from build123d import *

# Parameters (mm, degrees)
SKETCH_1_W          = 25
SKETCH_1_H          = 25
EXTRUDE_1_DEPTH     = 10
SKETCH_2_W          = 12.5
SKETCH_2_H          = 12.5
CUT_EXTRUDE_1_DEPTH = 21.310096012
SKETCH_3_W          = 25
SKETCH_3_H          = 25
EXTRUDE_2_DEPTH     = 5
SKETCH_4_R          = 2
CUT_EXTRUDE_2_DEPTH = 24.184046239
SKETCH_5_W          = 15
SKETCH_5_H          = 40
EXTRUDE_3_DEPTH     = 3
SKETCH_9_W          = 30
SKETCH_9_H          = 10
EXTRUDE_7_DEPTH     = 3
SKETCH_11_R         = 1.5
CUT_EXTRUDE_3_DEPTH = 50.749371855
EXTRUDE_8_DEPTH     = 12.5
EXTRUDE_9_DEPTH     = 3
SKETCH_15_R         = 1.25
CUT_EXTRUDE_4_DEPTH = 10
EXTRUDE_START       = -3
EXTRUDE_10_DEPTH    = 3


# Read off the part's stored shape, not the designer's step: 凸台-拉伸10
with BuildPart() as part:
    # 草图1 → 凸台-拉伸1 (new body)
    with BuildSketch(Plane.XY):
        Rectangle(SKETCH_1_W, SKETCH_1_H)
    extrude(amount=EXTRUDE_1_DEPTH)

    # 草图2 → 切除-拉伸1 (cut, through all)
    with BuildSketch(Plane.XY.offset(10)):
        Rectangle(SKETCH_2_W, SKETCH_2_H)
    extrude(amount=-CUT_EXTRUDE_1_DEPTH, mode=Mode.SUBTRACT)

    # 草图3 → 凸台-拉伸2 (add)
    with BuildSketch(Plane.XY.offset(10)):
        Rectangle(SKETCH_3_W, SKETCH_3_H)
    extrude(amount=EXTRUDE_2_DEPTH)

    # 草图4 → 切除-拉伸2 (cut, through all)
    with BuildSketch(Plane.XY.offset(15)):
        Circle(SKETCH_4_R)
    extrude(amount=-CUT_EXTRUDE_2_DEPTH, mode=Mode.SUBTRACT)

    # 草图5 → 凸台-拉伸3 (add)
    with BuildSketch(Plane(origin=(-12.5, 12.5, 0), x_dir=(0, 0, -1), z_dir=(0.7071067811865477, -0.7071067811865474, 0))):
        with Locations((-20, 0)):
            Rectangle(SKETCH_5_W, SKETCH_5_H)
    extrude(amount=EXTRUDE_3_DEPTH)

    # 草图9 → 凸台-拉伸7 (add)
    with BuildSketch(Plane(origin=(-10.378679656, 10.378679656, 0), x_dir=(0, 0, -1), z_dir=(0.7071067811865477, -0.7071067811865474, 0))):
        with Locations((-20, 25)):
            Rectangle(SKETCH_9_W, SKETCH_9_H)
    extrude_7 = extrude(amount=-EXTRUDE_7_DEPTH)

    # 草图11 → 切除-拉伸3 (cut, through all)
    with BuildSketch(Plane(origin=(-12.5, 12.5, 0), x_dir=(0, 0, 1), z_dir=(-0.7071067811865477, 0.7071067811865474, 0))):
        with Locations(Location((11, 24, 0), (0, 0, 270))):
            Circle(SKETCH_11_R)
        with Locations(Location((29, 24, 0), (0, 0, 270))):
            Circle(SKETCH_11_R)
    cut_extrude_3 = extrude(amount=-CUT_EXTRUDE_3_DEPTH, mode=Mode.SUBTRACT)

    # 草图12 → 凸台-拉伸8 (add)
    with BuildSketch(Plane(origin=(0, 0, 12.5), x_dir=(-1, 0, 0), z_dir=(0, 0, -1))):
        Polygon((8.257359313, 12.5), (12.5, 8.257359313), (14.621320344, 10.378679656), (10.378679656, 14.621320344), align=None)
    extrude(amount=EXTRUDE_8_DEPTH)

    # 草图13 → 凸台-拉伸9 (add)
    with BuildSketch(Plane(origin=(12.5, 12.5, 0), x_dir=(0, 0, -1), z_dir=(-0.7071067811865474, -0.7071067811865477, 0))):
        with BuildLine():
            Line((-27.5, -14.67766953), (-12.5, -14.67766953))
            ThreePointArc((-12.5, -14.67766953), (-3.210155108, -9.92766953), (0, 0))
            Line((0, 0), (-15, 0))
            ThreePointArc((-15, 0), (-18.349852274, -9.808698696), (-27.5, -14.67766953))
        make_face()
    extrude_9 = extrude(amount=EXTRUDE_9_DEPTH)

    # 草图15 → 切除-拉伸4 (cut)
    with BuildSketch(Plane(origin=(12.5, 0, 0), x_dir=(0, 0, -1), z_dir=(1, 0, 0))):
        with Locations(Location((-7.5, 0, 0), (0, 0, 90))):
            Circle(SKETCH_15_R)
    cut_extrude_4 = extrude(amount=-CUT_EXTRUDE_4_DEPTH, mode=Mode.SUBTRACT)

    # 凸台-拉伸10 outline → 凸台-拉伸10 (add)
    with BuildSketch(Plane(origin=(12.5, 12.5, 0), x_dir=(0, 0, -1), z_dir=(0.7071067811865474, 0.7071067811865477, 0)).offset(EXTRUDE_START)):
        with BuildLine():
            ThreePointArc((-12.5, 14.67766953), (-3.949281056, 10.728388475), (0, 2.177669532))
            Line((0, 2.177669532), (0, 17.67766953))
            Line((0, 17.67766953), (-12.5, 17.67766953))
            Line((-12.5, 17.67766953), (-12.5, 14.67766953))
        make_face()
    extrude_10 = extrude(amount=EXTRUDE_10_DEPTH)

    # 镜向3: 凸台-拉伸7, 切除-拉伸3, 凸台-拉伸9, 切除-拉伸4, 凸台-拉伸10 across plane
    add(extrude_7.mirror(Plane(origin=(0, 0, 0), x_dir=(0, 0, 1), z_dir=(-0.7071067811865474, -0.7071067811865477, 0))))
    add(cut_extrude_3.mirror(Plane(origin=(0, 0, 0), x_dir=(0, 0, 1), z_dir=(-0.7071067811865474, -0.7071067811865477, 0))), mode=Mode.SUBTRACT)
    add(extrude_9.mirror(Plane(origin=(0, 0, 0), x_dir=(0, 0, 1), z_dir=(-0.7071067811865474, -0.7071067811865477, 0))))
    add(cut_extrude_4.mirror(Plane(origin=(0, 0, 0), x_dir=(0, 0, 1), z_dir=(-0.7071067811865474, -0.7071067811865477, 0))), mode=Mode.SUBTRACT)
    add(extrude_10.mirror(Plane(origin=(0, 0, 0), x_dir=(0, 0, 1), z_dir=(-0.7071067811865474, -0.7071067811865477, 0))))


solid = part.part
Check sheet for the modelled part. Datum: model origin and axes. Units: mm. A direction names the side the tool comes from. Round coordinates to 2 decimals unless told otherwise and drop trailing zeros. Loops run counter-clockwise (first coordinate to the right, second up) from the corner with the lowest first, then second, coordinate; pieces in that order, holes last. Notation, with made-up numbers: (33, 79.25) - (68, 79.25) arc R30 cw to (68, 113.25) - close; hole circle Ø1 at (20.25, -31). An arc over 180 degrees is marked (long way). Answer as CSV lines item,"result". Start each with the question number.
Item 1: Release check for a two-part mould opening along Z. For faces 6 (the cylindrical face through (-12.235, -10.673, -0.044)), 7 (the flat face through (6.54, 27.3, 20.21)), 8 (the cylindrical face through (9.42, -0.27, 6.28)), 9 (the flat face through (-29, -6, 35)) record: +Z half, -Z half, draft (parallel to the pull), parting line (faces both ways), or undercut.
Item 2: Section check D-D (x = -23.5). Record the boundary of the cut face in (y, z), and give its area (3 significant figures).
Item 3: Set-up check for faces 1 (the flat face through (-32.638, -9.789, 20.21)), 2 (the flat face through (-27.3, -6.54, 20.21)), 3 (the flat face through (-25.567, -2.718, 8.802)), 4 (the flat face through (2.718, 25.567, 31.302)), 5 (the flat face through (-25.567, -2.718, 31.302)): record each of +Z, -Z, +X, -X, +Y, -Y from which the full face is reachable in a straight line by a thin tool's end or side.
Item 4: Scan lines: line 1 (X direction, y = -2.5, z = 13); line 2 (Y direction, x = -0.5, z = 11.5); line 3 (X direction, y = -10.75, z = 7.5). Record each from-to range of solid material in increasing order. Write a range as [from, to].
Item 5: Section check B-B (x = -4). Record the boundary of the cut face in (y, z), and give its area (3 significant figures).
Item 6: Section check A-A (z = 7.5). Count the separate pieces of the cut face and the enclosed holes in it, and give its area (3 significant figures).
Item 7: Depth check by flat-ended pin: P1, Ø8.5, axis at x = -17.5, y = 6.5, coming from the -Z side; P2, Ø2, axis at y = 0, z = 7.5, coming from the +X side; P3, Ø8, axis at x = -2.5, z = 3.5, coming from the +Y side; P4, Ø3, axis at x = 0, y = 0, coming from the +Z side. Enter the tip coordinate at first touch or a pass-through.
Report:
1,face 6,"-Z half"
1,face 7,"draft"
1,face 8,"undercut"
1,face 9,"+Z half"
2,outline,"(-2.74, 12.5) - (-1.5, 12.5) - (-1.5, 0) - (1.5, 0) - (1.5, 27.5) - (-2.74, 27.5) - close"
2,area,"101 mm2"
3,face 1,"+Z, -Z, -X, -Y"
3,face 2,"+Z, -Z, -Y"
3,face 3,"-Z"
3,face 4,"+Z, -X, -Y"
3,face 5,"+Z, +X, +Y"
4,line 1,"x = [-27.5, -23.26], [-22.5, -18.26], [-12.5, 12.5]"
4,line 2,"y = [-12.5, -1.94], [1.94, 12.5], [21.26, 24.5]"
4,line 3,"x = [-31.68, -31.51], [-14.25, -1.25], [1.25, 12.5]"
5,outline,"(-12.5, 0) - (-6.25, 0) - (-6.25, 10) - (6.25, 10) - (6.25, 0) - (12.5, 0) - (12.5, 15) - (-12.5, 15) - close; (16.76, 12.5) - (21, 12.5) - (21, 27.5) - (16.76, 27.5) - close"
5,area,"314 mm2"
6,separate pieces,"4"
6,enclosed holes,"0"
6,area,"604 mm2"
7,P1,"stops at z = 12.5"
7,P2,"stops at x = -6.25"
7,P3,"stops at y = 25"
7,P4,"passes through"
